Job drawing, mm, ordinate dimensions from the low corner. One solid piece. A direction names the side the tool comes from. Coordinates: 2 decimals unless noted, no trailing zeros. Loops run counter-clockwise (first coordinate to the right, second up) from the corner with the lowest first, then second, coordinate; pieces in that order, holes last. Notation, with made-up numbers: (85, 3) - (140, 3) arc R23 cw to (140, 42) - close; hole circle Ø11 at (80, 86.25). An arc over 180 degrees is marked (long way). Use a Markdown table: item, result. Add a question column.
1) Drop flat-ended pins along their axis: P1, Ø0.9, axis at y = 1.5, z = 13, coming from the +X side; P2, Ø3, axis at y = 3, z = 14, coming from the -X side; P3, Ø1.5, axis at x = 9.5, y = 2.5, coming from the -Z side. Give the stop position or say it passes through.
2) Pull direction Z, two halves, no side cores. Call the marked faces 1, 2 and 3: +Z half, -Z half, draft (parallel to the pull), parting line (faces both ways), or undercut.
3) Band-saw the part on D-D (x = 2). Give the cut face in (y, z).
4) Probe probe 1 along Z at (x, y) = (5, 4.6) (1 decimal); probe 2 along Y at (x, z) = (7.25, 2). List the from-to ranges inside material, lowest first. Write a range as [from, to].
5) Tool access for the marked faces 4, 5, 6, 7 and 8: list every direction of +Z, -Z, +X, -X, +Y, -Y with a clear straight run to the whole face (end or side of a thin tool).
6) Band-saw the part on A-A (z = 12). Give the cut face in (x, y).
7) Band-saw the part on B-B (x = 12). Give the cut face in (y, z).
8) Band-saw the part on C-C (y = 5.25). Give the number of separate pieces and of enclosed holes in the cut face, plus the area to 3 significant figures.
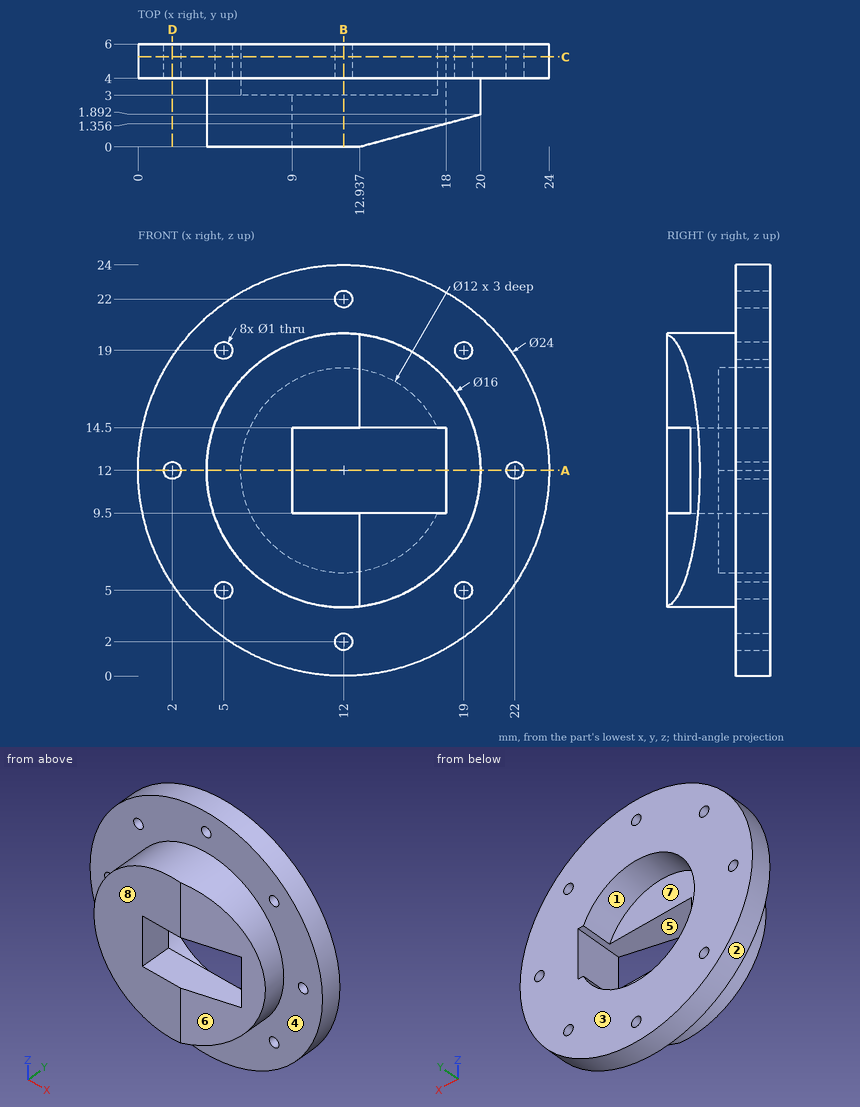
Answer block:
| question | item | result |
|---|---|---|
| 1 | P1 | x = 19.96 |
| 1 | P2 | x = 0.03 |
| 1 | P3 | z = 4.19 |
| 2 | face 1 | undercut |
| 2 | face 2 | parting line |
| 2 | face 3 | draft |
| 3 | outline | (4, 5.37) - (6, 5.37) - (6, 11.5) - (4, 11.5) - close; (4, 12.5) - (6, 12.5) - (6, 18.63) - (4, 18.63) - close |
| 4 | probe 1 | [2.3, 4.5], [5.5, 18.5], [19.5, 21.7] |
| 4 | probe 2 | [4, 6] |
| 5 | face 4 | -Y |
| 5 | face 5 | +Y, -Y |
| 5 | face 6 | +Z, -Z, +X, -Y |
| 5 | face 7 | +Y |
| 5 | face 8 | +Z, -Z, +X, -X, -Y |
| 6 | outline | (0, 4) - (1.5, 4) - (1.5, 6) - (0, 6) - close; (2.5, 4) - (4, 4) - (4, 0) - (9, 0) - (9, 3) - (6, 3) - (6, 6) - (2.5, 6) - close; (18, 1.36) - (20, 1.89) - (20, 4) - (21.5, 4) - (21.5, 6) - (18, 6) - close; (22.5, 4) - (24, 4) - (24, 6) - (22.5, 6) - close |
| 7 | outline | (0, 4) - (4, 4) - (4, 2.5) - (6, 2.5) - (6, 6) - (3, 6) - (3, 9.5) - (0, 9.5) - close; (0, 14.5) - (3, 14.5) - (3, 18) - (6, 18) - (6, 21.5) - (4, 21.5) - (4, 20) - (0, 20) - close; (4, 0) - (6, 0) - (6, 1.5) - (4, 1.5) - close; (4, 22.5) - (6, 22.5) - (6, 24) - (4, 24) - close |
| 8 | separate pieces | 1 |
| 8 | enclosed holes | 9 |
| 8 | area | 332 mm2 |
